The listing builds one solid part. Answer for the finished solid, in the listing's coordinates (mm). Face numbers are marked on the shaded views. A direction names the side the tool comes from. Give positions to 0.01 mm unless a question says otherwise; leave off trailing zeros. Write each loop counter-clockwise with the first axis right and the second up, starting at its lowest first coordinate (ties: lowest second). Pieces come first, ordered by that corner, then holes. Notation, with made-up numbers: (89.25, 59) - (96.25, 59) arc R22 ccw to (96.25, 72) - close; hole circle Ø3 at (-2.5, 17.25). An arc over 180 degrees is marked (long way). Return JSON: item names as keys, results as strings.
Autodesk Inventor part; units mm, degrees
ref_plane "YZ Plane" through (0, 0, 0) normal (1, 0, 0) x (0, 1, 0)
ref_plane "XZ Plane" through (0, 0, 0) normal (0, 1, 0) x (-1, 0, 0)
ref_plane "XY Plane" through (0, 0, 0) normal (0, 0, 1) x (1, 0, 0)
ref_plane "Arbeitsebene1" through (0, 0, 0) normal (0, 0, 1) x (1, 0, 0)
sketch "Skizze1" plane through (0, 0, 0) normal (0, 0, 1) x (1, 0, 0)
  line L0 (-43.5249, 65.0249) -> (-30, 65.0249)
  line L1 (-43.5249, -65.0249) -> (-43.5249, 65.0249)
  circle A0 centre (-50, 52.5) radius 1.4
  line L2 (-46, 72.5) -> (-50, 72.5)
  line L3 (-55, 67.5) -> (-55, 59.5)
  line L4 (-55, 44.5) -> (-51, 44.5)
  line L5 (-46, 49.5) -> (-46, 58.0276)
  line L6 (-55, 44.5) -> (-70, 44.5)
  line L7 (-70, 44.5) -> (-70, 54.5)
  line L8 (-70, 54.5) -> (-60, 54.5)
  line L9 (-55, 54.5) -> (-55, 44.5)
  circle A1 centre (-50, 52.5) radius 1.6
  arc A2 (-25.9255, 64.7266) -> (-46, 72.5) centre (-46, 42.6923) ccw
  arc A3 (-26.9357, 63.6178) -> (-30.5378, 66.404) centre (-46, 42.6923) ccw
  arc A4 (-30.5378, 66.404) -> (-46, 58.0276) centre (-36, 58.0276) ccw
  arc A5 (-26.9357, 63.6178) -> (-25.9255, 64.7266) centre (-26.4306, 64.1722) ccw
  arc A6 (-46, 58.0276) -> (-42.9999, 50.8861) centre (-36, 58.0276) ccw
  arc A7 (-46, 52.3487) -> (-44.0499, 49.8149) centre (-36, 58.0276) ccw
  arc A8 (-44.0499, 49.8149) -> (-42.9999, 50.8861) centre (-43.5249, 50.3505) ccw
  arc A9 (-51, 44.5) -> (-46, 49.5) centre (-51, 49.5) ccw
  arc A10 (-60, 54.5) -> (-55, 59.5) centre (-60, 59.5) ccw
  arc A11 (-50, 72.5) -> (-55, 67.5) centre (-50, 67.5) ccw
  point P0 (0, 0)
  point P1 (-55, 72.5)
  point P2 (-46, 44.5)
  point P3 (-27.3644, 64.0006)
  point P4 (-46, 71)
  dimension "d0" = 4
  dimension "d1" = 5
  dimension "d2" = 8
  dimension "d3" = 10
  dimension "d4" = 15
  dimension "d5" = 20
  dimension "d6" = 3.2
  dimension "d10" = 1.5
  dimension "d12" = 10
  dimension "d13" = 0.75
  dimension "d14" = 1.5
  dimension "d15" = 5
extrude "Extrusion1" add sketch "Skizze1" along normal blind 6 contours L1 A4 L5 A9 L4 L6 L7 L8 A10 L3 A11 L2 A2 A5 A3 L0 | L0 A4 L1 | A6 A8 L1 | L1 A8 A7 L5 A6
fillet "Rundung1" radius 2 3 edges at (-70, 54.5, 3) (-70, 44.5, 3) (-46, 72.5, 3)
sketch "Skizze2" plane through (0, 0, 0) normal (0, 0, -1) x (-1, 0, 0)
  line L0 (70, 52.5) -> (70, 46.5)
  arc A0 (68, 44.5) -> (70, 46.5) centre (68, 46.5) ccw
  line L1 (68, 44.5) -> (51, 44.5)
  arc A1 (46, 49.5) -> (51, 44.5) centre (51, 49.5) ccw
  line L2 (46, 49.5) -> (46, 52.3487)
  arc A2 (44.0499, 49.8149) -> (46, 52.3487) centre (36, 58.0276) ccw
  arc A3 (42.9999, 50.8861) -> (44.0499, 49.8149) centre (43.5249, 50.3505) ccw
  arc A4 (42.9999, 50.8861) -> (30.5378, 66.404) centre (36, 58.0276) ccw
  arc A5 (30.5378, 66.404) -> (26.9357, 63.6178) centre (46, 42.6923) ccw
  arc A6 (25.9255, 64.7266) -> (26.9357, 63.6178) centre (26.4306, 64.1722) ccw
  arc A7 (46, 72.5) -> (25.9255, 64.7266) centre (46, 42.6923) ccw
  line L3 (46, 72.5) -> (50, 72.5)
  arc A8 (55, 67.5) -> (50, 72.5) centre (50, 67.5) ccw
  line L4 (55, 67.5) -> (55, 59.5)
  arc A9 (55, 59.5) -> (60, 54.5) centre (60, 59.5) ccw
  line L5 (60, 54.5) -> (68, 54.5)
  arc A10 (70, 52.5) -> (68, 54.5) centre (68, 52.5) ccw
  line L6 (70, 52.5) -> (70, 46.5)
  circle A11 centre (50, 52.5) radius 1.6
  line L7 (64, 54.5) -> (64, 44.5)
  point P0 (0, 0)
  dimension "d16" = 6
extrude "Extrusion2" add sketch "Skizze2" along normal blind 5.5 contours L0 A0 L1 L7 L5 A10
sketch "Skizze3" plane through (-70, 46.5, 6) normal (-1, 0, 0) x (0, 0, 1)
  line L0 (0, 0) -> (-11.5, 0)
  line L1 (0, 6) -> (0, 0)
  line L2 (0, 6) -> (-11.5, 6)
  line L3 (-11.5, 0) -> (-11.5, 6)
  circle A0 centre (-8.4091, 3) radius 1.4
  point P0 (-6, -46.5)
  dimension "d19" = 2.8
extrude "Extrusion3" cut sketch "Skizze3" against normal through all contours A0
properties part number "30_xystage_gp-010b_adapter_multiwellplate_flexureclamp"
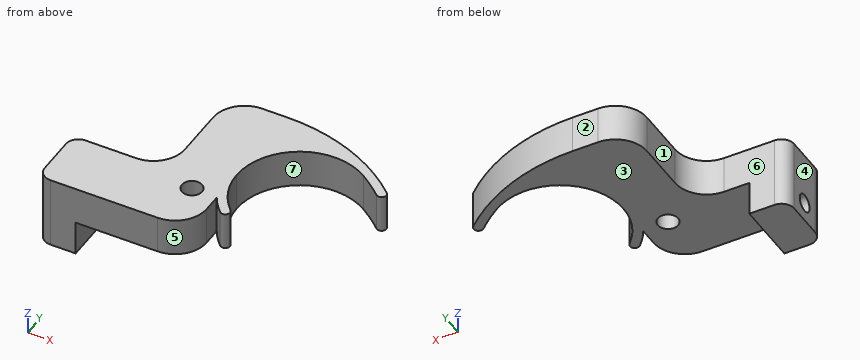
Item 1: A cutting plane is placed at C-C on z = -5. Determine the outline of the cut face in (x, y).
Answer below:
{"outline": "(-70, 46.5) arc R2 ccw to (-68, 44.5) - (-64, 44.5) - (-64, 54.5) - (-68, 54.5) arc R2 ccw to (-70, 52.5) - close"}
Item 2: Flat-ended cylindrical pins translate along their axes: P1, Ø3, axis at y = 49, z = -2, coming from the +X side; P2, Ø5, axis at y = 62, z = 2.5, coming from the -X side; P3, Ø0.9, axis at y = 51, z = 1.5, coming from the +X side. Find the tip coordinate at first contact, or state that the pin passes through.
Answer below:
{"P1": "stops at x = -64", "P2": "stops at x = -55", "P3": "stops at x = -42.8"}
Item 3: A cutting plane is placed at D-D on y = 46. Determine the outline of the cut face in (x, z), then the cut area to 3 significant figures.
Answer below:
{"outline": "(-69.94, -5.5) - (-64, -5.5) - (-64, 0) - (-47.43, 0) - (-47.43, 6) - (-69.94, 6) - close", "area": "168 mm²"}
Item 4: For the marked faces 1, 2 and 3, determine the directions among +Z, -Z, +X, -X, +Y, -Y from which every point of the face is accessible in a straight line to the end or side of a thin tool.
Answer below:
{"face 1": "+Z, -Z, -X, +Y", "face 2": "+Z, -Z, +X, -X, +Y", "face 3": "-Z, +X, +Y, -Y"}
Item 5: Consider L1, parallel to Z at x = -30.5, y = 66.75; L2, parallel to X at y = 64.75, z = 0.25; L3, parallel to Y at x = -65, z = 2.5. Determine where each line is inside the solid, lowest interval first.
Answer below:
{"L1": "z = 0 to 6", "L2": "x = -55 to -43.4, -28.26 to -25.95", "L3": "y = 44.5 to 54.5"}
Item 6: A cutting plane is placed at A-A on z = 1.5. Determine the outline of the cut face in (x, y).
Answer below:
{"outline": "(-70, 46.5) arc R2 ccw to (-68, 44.5) - (-51, 44.5) arc R5 ccw to (-46, 49.5) - (-46, 52.35) arc R11.5 ccw to (-44.05, 49.81) arc R0.75 ccw to (-43, 50.89) arc R10 cw to (-46, 58.03) arc R10 cw to (-30.54, 66.4) arc R28.31 cw to (-26.94, 63.62) arc R0.75 ccw to (-25.93, 64.73) arc R29.81 ccw to (-46, 72.5) - (-50, 72.5) arc R5 ccw to (-55, 67.5) - (-55, 59.5) arc R5 cw to (-60, 54.5) - (-68, 54.5) arc R2 ccw to (-70, 52.5) - close; hole circle Ø3.2 at (-50, 52.5)"}
Item 7: The mould has two halves that part along Y. Classify the marked faces 4, 5, 6 and 7: +Y half, -Y half, draft (parallel to the pull), parting line (faces both ways), or undercut.
Answer below:
{"face 4": "draft", "face 5": "-Y half", "face 6": "+Y half", "face 7": "undercut"}
Item 8: A cutting plane is placed at B-B on x = -49. Determine the outline of the cut face in (y, z), then the cut area to 3 significant figures.
Answer below:
{"outline": "(44.92, 0) - (51.25, 0) - (51.25, 6) - (44.92, 6) - close; (53.75, 0) - (72.5, 0) - (72.5, 6) - (53.75, 6) - close", "area": "151 mm²"}
